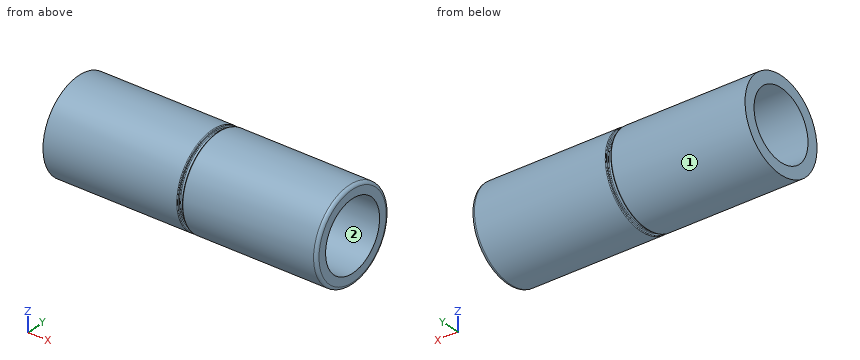
```python
from build123d import *

# Parameters (mm, degrees)
FILLET2_R = 0.2


with BuildPart() as part:
    # Sketch2 → Revolve1 (revolve)
    with BuildSketch(Plane(origin=(0, 0, 0), x_dir=(1, 0, 0), z_dir=(0, 1, 0))):
        with BuildLine():
            Line((18, 2.25), (18, 3))
            Line((18, 3), (9.2, 3))
            ThreePointArc((9.2, 3), (9.164644661, 2.985355339), (9.15, 2.95))
            Line((9.15, 2.95), (9.15, 2.85))
            ThreePointArc((9.15, 2.85), (9.135355339, 2.814644661), (9.1, 2.8))
            Line((9.1, 2.8), (8.9, 2.8))
            ThreePointArc((8.9, 2.8), (8.864644661, 2.814644661), (8.85, 2.85))
            Line((8.85, 2.85), (8.85, 2.95))
            ThreePointArc((8.85, 2.95), (8.835355339, 2.985355339), (8.8, 3))
            Line((8.8, 3), (0, 3))
            Line((0, 3), (0, 2.25))
            Line((0, 2.25), (18, 2.25))
        make_face()
    revolve(axis=Axis((0, 0, 0), (1, 0, 0)))

    # Fillet2
    fillet2_edges = [part.edges().sort_by_distance(p)[0] for p in [
        (18, 0, 3),
    ]]
    fillet(fillet2_edges, radius=FILLET2_R)


solid = part.part
```
Can you work these out from the model? Positions are in its coordinate system, mm. Face numbers are marked on the shaded views. Coordinates: 2 decimals unless noted, no trailing zeros. Loops run counter-clockwise (first coordinate to the right, second up) from the corner with the lowest first, then second, coordinate; pieces in that order, holes last.
1) I need wall thicknesses on probe 1 along Y at (x, z) = (10.5, 0); probe 2 along Y at (x, z) = (16.25, -2); probe 3 along Z at (x, y) = (8, 1.75). Which ranges of each line are inside material? Lowest first, please.
2) Imagine slicing it at A-A on y = 0. List the corners of the cut face in (x, z) for me.
3) Thinking about a two-plate mould opening in Y: for the marked faces 1 and 2, which applies, pulls with the +Y half, pulls with the -Y half, needs draft (parallel to the pull), parting line crosses it, or undercut?
4) Imagine slicing it at C-C on x = 6.5. List the corners of the cut face in (y, z) for me, plus the area to 3 significant figures.
5) For pin 1 (1 mm diameter, centred on x = 16, y = -2, fed in from +Z); pin 2 (2 mm diameter, centred on x = 6, z = 2, fed in from +Y), each with a flat end and sliding along its axis, tell me the tip position at first contact or that it passes through.
Completed:
1. probe 1: y = -3 to -2.25, 2.25 to 3
1. probe 2: y = -2.24 to -1.03, 1.03 to 2.24
1. probe 3: z = -2.44 to -1.41, 1.41 to 2.44
2. outline: (0, -3) - (8.8, -3) arc R0.05 ccw to (8.85, -2.95) - (8.85, -2.85) arc R0.05 cw to (8.9, -2.8) - (9.1, -2.8) arc R0.05 cw to (9.15, -2.85) - (9.15, -2.95) arc R0.05 ccw to (9.2, -3) - (17.8, -3) arc R0.2 ccw to (18, -2.8) - (18, -2.25) - (0, -2.25) - close; (0, 2.25) - (18, 2.25) - (18, 2.8) arc R0.2 ccw to (17.8, 3) - (9.2, 3) arc R0.05 ccw to (9.15, 2.95) - (9.15, 2.85) arc R0.05 cw to (9.1, 2.8) - (8.9, 2.8) arc R0.05 cw to (8.85, 2.85) - (8.85, 2.95) arc R0.05 ccw to (8.8, 3) - (0, 3) - close
3. face 1: parting line crosses it
3. face 2: undercut
4. outline: circle Ø6 at (0, 0); hole circle Ø4.5 at (0, 0)
4. area: 12.4 mm2
5. pin 1: stops at z = 2.6
5. pin 2: stops at y = 2.83
